For this review, use the dimensioned drawing (mm, ordinates from the lowest corner) and the shaded views. A direction names the side the tool comes from. Coordinates: 2 decimals unless noted, no trailing zeros. Loops run counter-clockwise (first coordinate to the right, second up) from the corner with the lowest first, then second, coordinate; pieces in that order, holes last. Notation, with made-up numbers: M 79.25,25 L 108.25,25 A16 cw 108.25,56 Z; hole C -20.5,63.5 d9. An arc over 180 degrees is marked long. One line per item, written item: value.
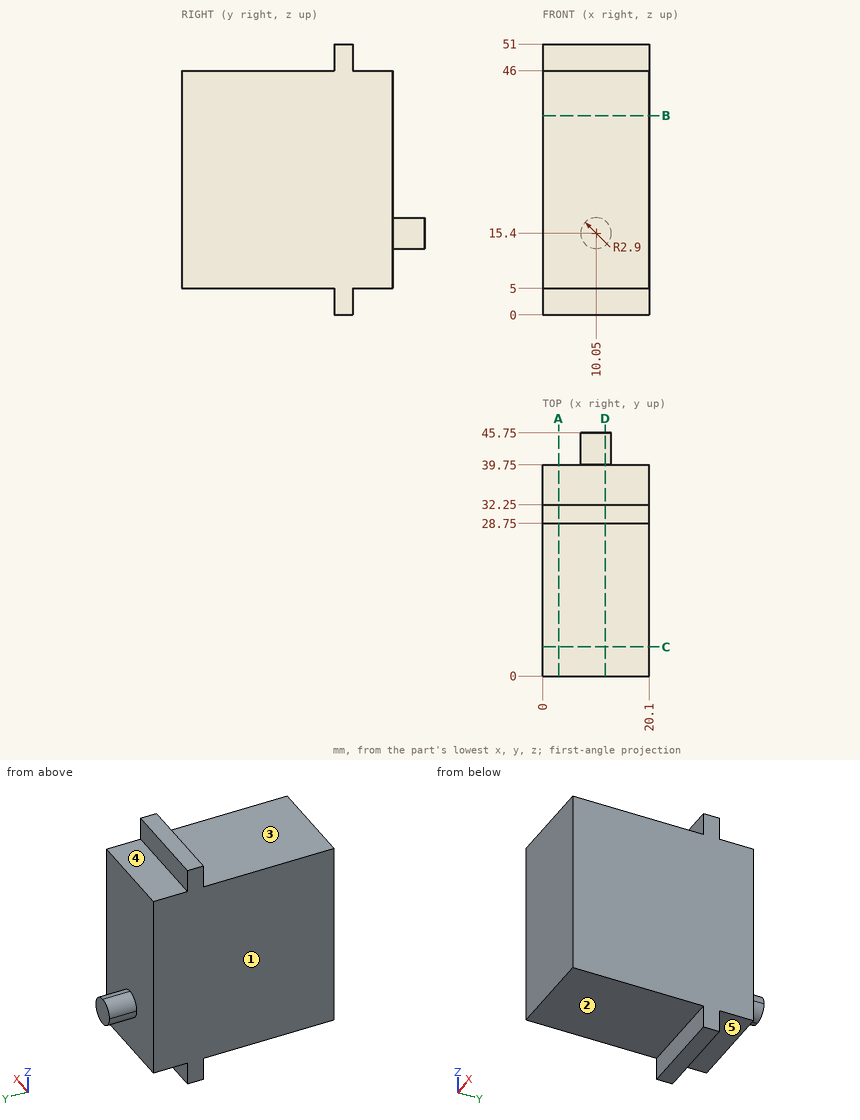
(1) Add section D-D on x = 11.75. State the section outline as (y, z) points.
Checks:
outline: M 0,5 L 28.75,5 L 28.75,0 L 32.25,0 L 32.25,5 L 39.75,5 L 39.75,13.05 L 45.75,13.05 L 45.75,17.75 L 39.75,17.75 L 39.75,46 L 32.25,46 L 32.25,51 L 28.75,51 L 28.75,46 L 0,46 Z
(2) Tool access review of the marked faces 1, 2, 3, 4 and 5: name each direction out of +Z, -Z, +X, -X, +Y, -Y from which nothing blocks a thin tool from reaching the whole face with its end or side.
Checks:
face 1: +Z, -Z, -X, +Y, -Y
face 2: -Z, +X, -X, -Y
face 3: +Z, +X, -X, -Y
face 4: +Z, +X, -X, +Y
face 5: -Z, +X, -X, +Y
(3) Add section A-A on x = 3. State the section outline as (y, z) points.
Checks:
outline: M 0,5 L 28.75,5 L 28.75,0 L 32.25,0 L 32.25,5 L 39.75,5 L 39.75,46 L 32.25,46 L 32.25,51 L 28.75,51 L 28.75,46 L 0,46 Z
(4) To check wall thickness, follow L1, parallel to Y at x = 10.25, z = 47; L2, parallel to Z at x = 2.75, y = 25.5; L3, parallel to Y at x = 5.75, z = 45. State the ranges of each line that lie inside material, in increasing order. Write a range as [from, to].
Checks:
L1: [28.75, 32.25]
L2: [5, 46]
L3: [0, 39.75]
(5) Insertion check: pin 1 Ø8 at (x, z) = (9.5, 19) entering from -Y; pin 2 Ø10 at (x, y) = (14, 19) entering from +Z; pin 3 Ø6 at (x, z) = (7.5, 10) entering from +Y; pin 4 Ø2.5 at (x, z) = (14.5, 3) entering from -Y. Each pin has a flat end and moves straight along its axis. Give the tip position at first contact, or say it passes through.
Checks:
pin 1: y = 0
pin 2: z = 46
pin 3: y = 39.75
pin 4: y = 28.75
(6) Add section C-C on y = 5.5. State the section outline as (x, z) points, then the cut area to 3 significant figures.
Checks:
outline: M 0,5 L 20.1,5 L 20.1,46 L 0,46 Z
area: 824 mm^2
(7) Add section B-B on z = 37.5. State the section outline as (x, y) points, then the cut area to 3 significant figures.
Checks:
outline: M 0,0 L 20.1,0 L 20.1,39.75 L 0,39.75 Z
area: 799 mm^2
